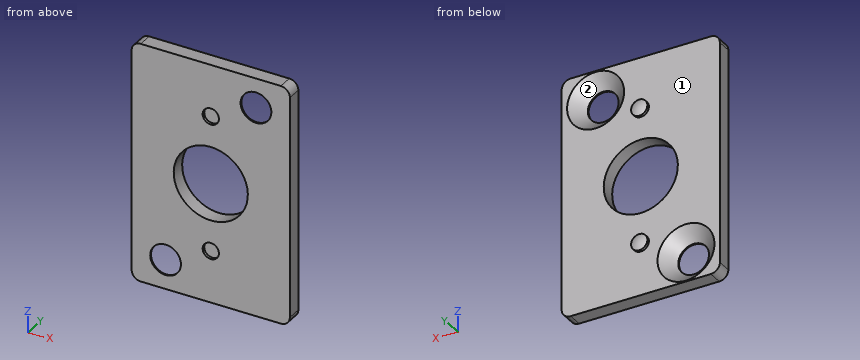
```python
from build123d import *

# Parameters (mm, degrees)
BASES_W                                         = 17.5
BASES_H                                         = 26.5
BASE_DEPTH                                      = 1.6
CSK_FOR_M3_FLAT_HEAD_MACHINE_SCREW1_D           = 3.4
CSK_FOR_M3_FLAT_HEAD_MACHINE_SCREW1_DEPTH       = 11
CSK_FOR_M3_FLAT_HEAD_MACHINE_SCREW1_CSINK_D     = 6.3
CSK_FOR_M3_FLAT_HEAD_MACHINE_SCREW1_CSINK_ANGLE = 90
CSK_FOR_M3_FLAT_HEAD_MACHINE_SCREW1_TIP         = 1.021463052
BORES_R                                         = 4.1
BORE_DEPTH                                      = 16.958853342
LOCKINGFEATURES_R                               = 0.9
LOCKING_FEATURE_DEPTH                           = 0.3
LF_DOME_FACE_RADIUS                             = 0.9
LF_DOME_HEIGHT                                  = 0.2
LF_HM_COPY_1_FACE_RADIUS                        = 0.9
LF_HM_COPY_1_HEIGHT                             = 0.2
LFBOTTOMCUT_R                                   = 0.9
LF_BOTTOM_CUT_DEPTH                             = 0.3
BASE_FILLET_R                                   = 1


with BuildPart() as part:
    # BaseS → BASE (new body)
    with BuildSketch(Plane(origin=(0, 0, 0), x_dir=(1, 0, 0), z_dir=(0, 1, 0))):
        Rectangle(BASES_W, BASES_H)
    extrude(amount=-BASE_DEPTH)

    # CSK for M3 Flat Head Machine Screw1
    with Locations(Plane(origin=(0, 0, 0), x_dir=(1, 0, 0), z_dir=(0, 1, 0))):
        with Locations((-5, 10), (5, -10)):
            CounterSinkHole(CSK_FOR_M3_FLAT_HEAD_MACHINE_SCREW1_D / 2, CSK_FOR_M3_FLAT_HEAD_MACHINE_SCREW1_CSINK_D / 2, depth=CSK_FOR_M3_FLAT_HEAD_MACHINE_SCREW1_DEPTH, counter_sink_angle=CSK_FOR_M3_FLAT_HEAD_MACHINE_SCREW1_CSINK_ANGLE)
            with Locations((0, 0, -(CSK_FOR_M3_FLAT_HEAD_MACHINE_SCREW1_DEPTH + CSK_FOR_M3_FLAT_HEAD_MACHINE_SCREW1_TIP / 2))):  # 118° drill point
                Cone(0, CSK_FOR_M3_FLAT_HEAD_MACHINE_SCREW1_D / 2, CSK_FOR_M3_FLAT_HEAD_MACHINE_SCREW1_TIP, mode=Mode.SUBTRACT)

    # BoreS → BORE (cut, through all)
    with BuildSketch(Plane(origin=(0, 0, 0), x_dir=(1, 0, 0), z_dir=(0, 1, 0))):
        with Locations(Location((0, 0, 0), (0, 0, 270))):
            Circle(BORES_R)
    extrude(amount=-BORE_DEPTH, mode=Mode.SUBTRACT)

    # LockingFeatureS → LOCKING FEATURE (add)
    with BuildSketch(Plane(origin=(0, 0, 0), x_dir=(1, 0, 0), z_dir=(0, 1, 0))):
        with Locations(Location((0, 7.5, 0), (0, 0, 270))):
            Circle(LOCKINGFEATURES_R)
    locking_feature = extrude(amount=LOCKING_FEATURE_DEPTH)

    # LF DOME: a dome of height H over a round flat face of radius A is a cap of a sphere of radius (A * A + H * H) / (2 * H)
    lf_dome_r = (LF_DOME_FACE_RADIUS * LF_DOME_FACE_RADIUS + LF_DOME_HEIGHT * LF_DOME_HEIGHT) / (2 * LF_DOME_HEIGHT)
    lf_dome_base = Plane((0, 0.3, -7.5), z_dir=(0, 1, 0))
    with Locations(lf_dome_base.offset(LF_DOME_HEIGHT - lf_dome_r)):
        lf_dome_ball = Sphere(lf_dome_r, mode=Mode.PRIVATE)
    add(split(lf_dome_ball, bisect_by=lf_dome_base, keep=Keep.TOP, mode=Mode.PRIVATE))

    # LF HM: LOCKING FEATURE across plane
    add(locking_feature.mirror(Plane.XY))

    # LF HM copy 1: a dome of height H over a round flat face of radius A is a cap of a sphere of radius (A * A + H * H) / (2 * H)
    lf_hm_copy_1_r = (LF_HM_COPY_1_FACE_RADIUS * LF_HM_COPY_1_FACE_RADIUS + LF_HM_COPY_1_HEIGHT * LF_HM_COPY_1_HEIGHT) / (2 * LF_HM_COPY_1_HEIGHT)
    lf_hm_copy_1_base = Plane((0, 0.3, 7.5), z_dir=(0, 1, 0))
    with Locations(lf_hm_copy_1_base.offset(LF_HM_COPY_1_HEIGHT - lf_hm_copy_1_r)):
        lf_hm_copy_1_ball = Sphere(lf_hm_copy_1_r, mode=Mode.PRIVATE)
    add(split(lf_hm_copy_1_ball, bisect_by=lf_hm_copy_1_base, keep=Keep.TOP, mode=Mode.PRIVATE))

    # LFBottomCut → LF BOTTOM CUT (cut)
    with BuildSketch(Plane(origin=(0, -1.6, 0), x_dir=(-1, 0, 0), z_dir=(0, -1, 0))):
        with Locations(Location((0, 7.5, 0), (0, 0, 270))):
            Circle(LFBOTTOMCUT_R)
        with Locations(Location((0, -7.5, 0), (0, 0, 90))):
            Circle(LFBOTTOMCUT_R)
    extrude(amount=-LF_BOTTOM_CUT_DEPTH, mode=Mode.SUBTRACT)

    # BASE FILLET
    base_fillet_edges = [part.edges().sort_by_distance(p)[0] for p in [
        (8.75, -0.8, 13.25),
        (-8.75, -0.8, 13.25),
        (-8.75, -0.8, -13.25),
        (8.75, -0.8, -13.25),
    ]]
    fillet(base_fillet_edges, radius=BASE_FILLET_R)


solid = part.part
```
Input: part model. Units: mm. Frame: model coordinates. Face numbers are marked on the shaded views. Give positions to 0.01 mm unless a question says otherwise; leave off trailing zeros. Loops run counter-clockwise (first coordinate to the right, second up) from the corner with the lowest first, then second, coordinate; pieces in that order, holes last.
1) Section query D-D on z = 5.5. Return the cut outline in (x, y), and give its area (3 significant figures).
A:
outline: (-8.75, -1.6) - (8.75, -1.6) - (8.75, 0) - (-8.75, 0) - close
area: 28.0 mm2
2) Section query A-A on z = 10. Return the cut outline in (x, y), and give its area (3 significant figures).
A:
outline: (-8.75, -1.6) - (3.3, -1.6) - (3.3, -1.45) - (1.85, 0) - (-8.75, 0) - close; (6.7, -1.6) - (8.75, -1.6) - (8.75, 0) - (8.15, 0) - (6.7, -1.45) - close
area: 20.5 mm2
3) Line query: L1, parallel to X at y = -1.5, z = -10; L2, parallel to X at y = -1.4, z = -7.5; L3, parallel to Z at x = -5, y = -1.5. Output: solid intervals per line, ascending.
A:
L1: x = -8.75 to -6.7, -3.3 to 8.75
L2: x = -8.75 to -0.9, 0.9 to 8.75
L3: z = -13.25 to -11.7, -8.3 to 13.25
4) Contact query for flat-ended pins moving along their axis: pin 1 (0.9 mm diameter, centred on x = -0.5, z = 8, fed in from -Y); pin 2 (3 mm diameter, centred on x = 5, z = 10, fed in from -Y); pin 3 (5 mm diameter, centred on x = 3.5, z = -3, fed in from +Y). Output: stop coordinate, or through.
A:
pin 1: stops at y = -1.6
pin 2: passes through
pin 3: stops at y = 0
5) Mould query, pull axis X, two halves, no side actions, for the marked faces 1 and 2. Classes: released by +X, released by -X, zero draft, split by the parting line, or undercut.
A:
face 1: zero draft
face 2: undercut
6) Section query B-B on x = 5. Return the cut outline in (y, z), and give its area (3 significant figures).
A:
outline: (-1.6, -13.25) - (0, -13.25) - (0, 6.85) - (-1.45, 8.3) - (-1.6, 8.3) - close; (-1.6, 11.7) - (-1.45, 11.7) - (0, 13.15) - (0, 13.25) - (-1.6, 13.25) - close
area: 34.9 mm2
7) Section query C-C on y = -0.75. Return the cut outline in (x, z).
A:
outline: (-8.75, -12.25) arc R1 ccw to (-7.75, -13.25) - (7.75, -13.25) arc R1 ccw to (8.75, -12.25) - (8.75, 12.25) arc R1 ccw to (7.75, 13.25) - (-7.75, 13.25) arc R1 ccw to (-8.75, 12.25) - close; hole circle Ø4.8 at (-5, -10); hole circle Ø8.2 at (0, 0); hole circle Ø4.8 at (5, 10)
